from build123d import *

# Parameters (mm, degrees)
F0_W     = 304.8
F0_H     = 203.2
F0_R     = 12.7
F1_DEPTH = 76.2
F2_W     = 152.4
F2_H     = 12.7
F3_DEPTH = 25.4
F4_W     = 50.8
F4_H     = 31.75
F5_DEPTH = 6.35


with BuildPart() as f1:
    # F0 (on Top) → F1 (new body)
    with BuildSketch(Plane.XY):
        Rectangle(F0_W, F0_H)
        with Locations((-127, -76.2)):
            Circle(F0_R, mode=Mode.SUBTRACT)
        with Locations((-63.5, -76.2)):
            Circle(F0_R, mode=Mode.SUBTRACT)
        with BuildLine():
            ThreePointArc((-127, -12.7), (-118.0197438789, -16.4197438789), (-114.3, -25.4))
            ThreePointArc((-114.3, -25.4), (-135.9802561211, -34.3802561211), (-127, -12.7))
        make_face(mode=Mode.SUBTRACT)
        with Locations((-63.5, -25.4)):
            Circle(F0_R, mode=Mode.SUBTRACT)
        with Locations((0, -76.2)):
            Circle(F0_R, mode=Mode.SUBTRACT)
        with Locations((63.5, -76.2)):
            Circle(F0_R, mode=Mode.SUBTRACT)
        with Locations((127, -76.2)):
            Circle(F0_R, mode=Mode.SUBTRACT)
        with Locations((0, -25.4)):
            Circle(F0_R, mode=Mode.SUBTRACT)
        with Locations((63.5, -25.4)):
            Circle(F0_R, mode=Mode.SUBTRACT)
        with Locations((127, -25.4)):
            Circle(F0_R, mode=Mode.SUBTRACT)
        with BuildLine():
            ThreePointArc((-114.3, 25.4), (-118.0197438789, 16.4197438789), (-127, 12.7))
            ThreePointArc((-127, 12.7), (-135.9802561211, 34.3802561211), (-114.3, 25.4))
        make_face(mode=Mode.SUBTRACT)
        with Locations((-63.5, 25.4)):
            Circle(F0_R, mode=Mode.SUBTRACT)
        with Locations((-127, 76.2)):
            Circle(F0_R, mode=Mode.SUBTRACT)
        with Locations((-63.5, 76.2)):
            Circle(F0_R, mode=Mode.SUBTRACT)
        with Locations((0, 25.4)):
            Circle(F0_R, mode=Mode.SUBTRACT)
        with Locations((63.5, 25.4)):
            Circle(F0_R, mode=Mode.SUBTRACT)
        with Locations((127, 25.4)):
            Circle(F0_R, mode=Mode.SUBTRACT)
        with Locations((0, 76.2)):
            Circle(F0_R, mode=Mode.SUBTRACT)
        with Locations((63.5, 76.2)):
            Circle(F0_R, mode=Mode.SUBTRACT)
        with Locations((127, 76.2)):
            Circle(F0_R, mode=Mode.SUBTRACT)
    extrude(amount=F1_DEPTH)

    # F2 (on face) → F3 (join)
    with BuildSketch(Plane(origin=(0, 0, 0), x_dir=(1, 0, 0), z_dir=(0, 0, -1))):
        Rectangle(F2_W, F2_H)
    extrude(amount=F3_DEPTH)

    # F4 (on face) → F5 (cut)
    with BuildSketch(Plane.XY.offset(76.2)):
        with Locations((-127, 66.675)):
            Rectangle(F4_W, F4_H)
        with Locations((-127, -66.675)):
            Rectangle(F4_W, F4_H)
        with Locations((127, 66.675)):
            Rectangle(F4_W, F4_H)
        with Locations((127, -66.675)):
            Rectangle(F4_W, F4_H)
    extrude(amount=-F5_DEPTH, mode=Mode.SUBTRACT)


solid = f1.part
Read the model definition and answer for the solid it produces. Units are mm, in the model's axes. A direction names the side the tool comes from. Coordinates: 2 decimals unless noted, no trailing zeros. Write each loop counter-clockwise with the first axis right and the second up, starting at its lowest first coordinate (ties: lowest second). Pieces come first, ordered by that corner, then holes. Notation, with made-up numbers: (40.25, -19) -> (65.25, -19) arc R23 cw to (65.25, 12) -> close; hole circle Ø9 at (66, 51). An arc over 180 degrees is marked (long way). Return JSON: item names as keys, results as strings.
(1) The part is cut by section B-B on y = 76.2. Give the vertices of the cut face in (x, z), then the cut area to 3 significant figures.
Answers below:
{"outline": "(-152.4, 0) -> (-139.7, 0) -> (-139.7, 69.85) -> (-152.4, 69.85) -> close; (-114.3, 0) -> (-76.2, 0) -> (-76.2, 76.2) -> (-101.6, 76.2) -> (-101.6, 69.85) -> (-114.3, 69.85) -> close; (-50.8, 0) -> (-12.7, 0) -> (-12.7, 76.2) -> (-50.8, 76.2) -> close; (12.7, 0) -> (50.8, 0) -> (50.8, 76.2) -> (12.7, 76.2) -> close; (76.2, 0) -> (114.3, 0) -> (114.3, 69.85) -> (101.6, 69.85) -> (101.6, 76.2) -> (76.2, 76.2) -> close; (139.7, 0) -> (152.4, 0) -> (152.4, 69.85) -> (139.7, 69.85) -> close", "area": "13,200 mm^2"}
(2) The part is cut by section A-A on x = -63.5. Give the vertices of the cut face in (y, z).
Answers below:
{"outline": "(-101.6, 0) -> (-88.9, 0) -> (-88.9, 76.2) -> (-101.6, 76.2) -> close; (-63.5, 0) -> (-38.1, 0) -> (-38.1, 76.2) -> (-63.5, 76.2) -> close; (-12.7, 0) -> (-6.35, 0) -> (-6.35, -25.4) -> (6.35, -25.4) -> (6.35, 0) -> (12.7, 0) -> (12.7, 76.2) -> (-12.7, 76.2) -> close; (38.1, 0) -> (63.5, 0) -> (63.5, 76.2) -> (38.1, 76.2) -> close; (88.9, 0) -> (101.6, 0) -> (101.6, 76.2) -> (88.9, 76.2) -> close"}
(3) Each of these flat-tipped pins is pushed along its axis until it touches: P1, Ø9.5, axis at x = -138.5, y = -68, coming from the +Z side; P2, Ø7.5, axis at x = -2, z = -16.5, coming from the -Y side. Where does it stop, or does it pass through?
Answers below:
{"P1": "z = 69.85", "P2": "y = -6.35"}
(4) For a pull along X with two mould halves and no side action, classify faces 5 (the flat face through (127, 63, 69.85)), 6 (the flat face through (-101.6, 66, 73)), 7 (the cylindrical face through (-57.64, 64.933, 37.567)) as pulls with the +X half, pulls with the -X half, needs draft (parallel to the pull), parting line crosses it, or undercut.
Answers below:
{"face 5": "needs draft", "face 6": "pulls with the -X half", "face 7": "undercut"}
(5) Which of the six approach directions +Z, -Z, +X, -X, +Y, -Y give full straight-line access (tool end or side, diameter ignored) to faces 1 (the flat face through (76.2, 0, -13)), 2 (the flat face through (-127, -63, 69.85)), 3 (the flat face through (101.6, 66, 73)), 4 (the cylindrical face through (70.327, 36.109, 37.567))?
Answers below:
{"face 1": "-Z, +X, +Y, -Y", "face 2": "+Z, -X", "face 3": "+Z, +X", "face 4": "+Z, -Z"}
(6) The part is cut by section D-D on x = 36. Give the vertices of the cut face in (y, z), then the cut area to 3 significant figures.
Answers below:
{"outline": "(-101.6, 0) -> (-6.35, 0) -> (-6.35, -25.4) -> (6.35, -25.4) -> (6.35, 0) -> (101.6, 0) -> (101.6, 76.2) -> (-101.6, 76.2) -> close", "area": "15,800 mm^2"}
(7) The part is cut by section C-C on z = 41. State how many separate pieces and enclosed holes the cut face has, then the cut area to 3 significant figures.
Answers below:
{"separate pieces": "1", "enclosed holes": "20", "area": "51,800 mm^2"}
(8) Consider line 1 along X through (y, z) = (-25, 44); line 2 along Y through (x, z) = (0, 33); line 3 along X through (y, z) = (-18, 70.5). Determine where each line is inside the solid, lowest interval first. Write a range as from..to.
Answers below:
{"line 1": "-152.4..-139.69, -114.31..-76.19, -50.81..-12.69, 12.69..50.81, 76.19..114.31, 139.69..152.4", "line 2": "-101.6..-88.9, -63.5..-38.1, -12.7..12.7, 38.1..63.5, 88.9..101.6", "line 3": "-152.4..-137.32, -116.68..-73.82, -53.18..-10.32, 10.32..53.18, 73.82..116.68, 137.32..152.4"}
